```python
from build123d import *

# Parameters (mm, degrees)
F0_W           = 101.6
F0_H           = 50.8
F1_DEPTH       = 12.7
F3_D           = 3.175
F3_CBORE_D     = 6.35
F3_CBORE_DEPTH = 6.35
F4_W           = 101.6
F4_H           = 25.4
F5_DEPTH       = 3.175
F6_SIZE        = 1.5875
F8_DEPTH       = 101.601


with BuildPart() as f1:
    # F0 (on Front) → F1 (new body)
    with BuildSketch(Plane.XZ):
        with Locations((6.362615, 4.069407)):
            Rectangle(F0_W, F0_H)
    extrude(amount=F1_DEPTH)

    # F3 (through all)
    with Locations(Plane.XZ.offset(12.7)):
        with Locations((-38.087385, -14.980593), (50.812615, -14.980593), (50.812615, 23.119407), (-38.087385, 23.119407)):
            CounterBoreHole(F3_D / 2, F3_CBORE_D / 2, F3_CBORE_DEPTH)

    # F4 (on face) → F5 (cut)
    with BuildSketch(Plane.XZ.offset(12.7)):
        with Locations((6.362615, 4.069407)):
            Rectangle(F4_W, F4_H)
    extrude(amount=-F5_DEPTH, mode=Mode.SUBTRACT)

    # F6
    f6_edges = [f1.edges().sort_by_distance(p)[0] for p in [
        (6.362615, -12.7, 29.469407),
        (6.362615, -12.7, -21.330593),
    ]]
    chamfer(f6_edges, length=F6_SIZE)

    # F7 (on face) → F8 (cut, through all)
    with BuildSketch(Plane.YZ.offset(57.162615)):
        Polygon((-5.34251, 16.769407), (-5.34251, -8.630593), (0, -3.288082), (0, 11.426897), align=None)
    extrude(amount=-F8_DEPTH, mode=Mode.SUBTRACT)


solid = f1.part
```
Source: CAD feature listing. Evaluate the final solid. Frame: model axes, mm. A direction names the side the tool comes from. Round coordinates to 2 decimals unless told otherwise and drop trailing zeros. Loops run counter-clockwise (first coordinate to the right, second up) from the corner with the lowest first, then second, coordinate; pieces in that order, holes last.
1. Section query B-B on x = 50.5. Give the number of separate pieces and of enclosed holes in the cut face, and give its area (3 significant figures).
2. Section query A-A on y = -1.75. Output: boundary loops of the cut face in (x, z) (1 decimal).
3. Access query for faces 1 (the flat face through (6, -12.7, 22)), 2 (the cylindrical face through (-35.06, -9.57, 24.07)), 3 (the flat face through (7, -5.343, 4)), 4 (the flat face through (6, -11, -8.631)). Directions: +Z, -Z, +X, -X, +Y, -Y. A direction counts if a zero-diameter tool reaches every point of the face in a straight line with its end or side. Return the directions, or none.
4. Mould query, pull axis Y, two halves, no side actions, for faces 5 (the flat face through (57.163, -6, 4)), 6 (the flat face through (7.07, -2.71, -6)), 7 (the flat face through (49, -6.35, -16)). Classes: released by +Y, released by -Y, zero draft, split by the parting line, or undercut.
5. Section query D-D on x = 17. Output: boundary loops of the cut face in (y, z) (1 decimal).
6. Section query C-C on z = 13. Output: boundary loops of the cut face in (x, y) (3 decimals), and give its area (3 significant figures).
7. Ray query, L1, parallel to Z at x = 49.5, y = -0.25; L2, parallel to Y at x = 51.5, z = 1 (3 decimals); L3, parallel to Z at x = -17, y = -4.5. Return the intervals inside material, ascending.
8. Contact query for flat-ended pins moving along their axis: pin 1 (5 mm diameter, centred on x = 51, z = -15.5, fed in from -Y); pin 2 (12.5 mm diameter, centred on x = 0, z = 9.5, fed in from -Y) (3 decimals); pin 3 (12.5 mm diameter, centred on x = 18, z = 5, fed in from +Y). Output: stop coordinate, or through.
Answers below:
1. separate pieces: 3
1. enclosed holes: 0
1. area: 335 mm2
2. outline: (-44.4, -21.3) - (57.2, -21.3) - (57.2, -5) - (-44.4, -5) - close; (-44.4, 13.2) - (57.2, 13.2) - (57.2, 29.5) - (-44.4, 29.5) - close; hole circle Ø3.2 at (-38.1, -15); hole circle Ø3.2 at (-38.1, 23.1); hole circle Ø3.2 at (50.8, -15); hole circle Ø3.2 at (50.8, 23.1)
3. face 1: +Z, -Z, +X, -X, -Y
3. face 2: -Y
3. face 3: +X, -X
3. face 4: +X, -X, -Y
4. face 5: zero draft
4. face 6: undercut
4. face 7: released by -Y
5. outline: (-12.7, -19.7) - (-11.1, -21.3) - (0, -21.3) - (0, -3.3) - (-5.3, -8.6) - (-5.3, 16.8) - (0, 11.4) - (0, 29.5) - (-11.1, 29.5) - (-12.7, 27.9) - (-12.7, 16.8) - (-9.5, 16.8) - (-9.5, -8.6) - (-12.7, -8.6) - close
6. outline: (-44.437, -9.525) - (57.163, -9.525) - (57.163, -5.343) - (-44.437, -5.343) - close; (-44.437, -1.573) - (57.163, -1.573) - (57.163, 0) - (-44.437, 0) - close
6. area: 585 mm2
7. L1: z = -21.33 to -15.87, -14.09 to -3.54, 11.68 to 22.23, 24.01 to 29.47
7. L2: y = -9.525 to -5.343
7. L3: z = -21.33 to -7.79, 15.93 to 29.47
8. pin 1: stops at y = -6.35
8. pin 2: stops at y = -9.525
8. pin 3: stops at y = -5.34
